```python
from build123d import *

# Parameters (mm, degrees)
RESSALTO_EXTRUS_O2_DEPTH = 20


with BuildPart() as part:
    # Esboço1 → Ressalto-extrusão2 (new body)
    with BuildSketch(Plane.XY):
        Polygon((0, 0), (0, 65), (50, 65), (50, 40), (85, 40), (85, 0), align=None)
    extrude(amount=-RESSALTO_EXTRUS_O2_DEPTH)


solid = part.part
```
Input: part model. Units: mm. Frame: model coordinates. A direction names the side the tool comes from. Give positions to 0.01 mm unless a question says otherwise; leave off trailing zeros. Order: outer loops, then holes, each group sorted by start corner. A loop starts at its lowest first (then second) coordinate and runs counter-clockwise, first axis right, second up. Notation, with made-up numbers: (44.25, 61) - (79.25, 61) arc R31 ccw to (79.25, 96) - close; hole circle Ø10 at (59, 17). An arc over 180 degrees is marked (long way). One line per item, written item: value.
1. Pin query (flat end, axial travel): pin 1 Ø10 at (x, z) = (75, -10) entering from +Y; pin 2 Ø10 at (y, z) = (57.5, -15) entering from +X. Return the tip coordinate at first contact, or that it passes through.
Determined:
pin 1: y = 40
pin 2: x = 50
2. Cut plane C-C, the plane y = 41. Output: boundary loops of the cut face in (x, z).
Determined:
outline: (0, -20) - (50, -20) - (50, 0) - (0, 0) - close
3. Line query: probe 1 along X at (y, z) = (41, -6.25); probe 2 along Y at (x, z) = (69, -16). Output: solid intervals per line, ascending.
Determined:
probe 1: 0 to 50
probe 2: 0 to 40
4. Reachability of faces 1 (the face through (67, 40, -10)), 2 (the face through (85, 20, -10)) from +Z, -Z, +X, -X, +Y, -Y: full face, straight path, thin tool, end or side. Return the list, or none.
Determined:
face 1: +Z, -Z, +X, +Y
face 2: +Z, -Z, +X, +Y, -Y
5. Cut plane B-B, the plane x = 78. Output: boundary loops of the cut face in (y, z), and give its area (3 significant figures).
Determined:
outline: (0, -20) - (40, -20) - (40, 0) - (0, 0) - close
area: 800 mm2
6. Cut plane A-A, the plane z = -12.25. Output: boundary loops of the cut face in (x, y).
Determined:
outline: (0, 0) - (85, 0) - (85, 40) - (50, 40) - (50, 65) - (0, 65) - close
